Check sheet for the modelled part. Datum: model origin and axes. Units: mm. Face numbers are marked on the shaded views. Round coordinates to 2 decimals unless told otherwise and drop trailing zeros. Write each loop counter-clockwise with the first axis right and the second up, starting at its lowest first coordinate (ties: lowest second). Pieces come first, ordered by that corner, then holes. Notation, with made-up numbers: (62, -27.75) -> (110, -27.75) arc R17 ccw to (110, -2.75) -> close; hole circle Ø10 at (51.25, 13). An arc over 180 degrees is marked (long way). One line per item, written item: value.
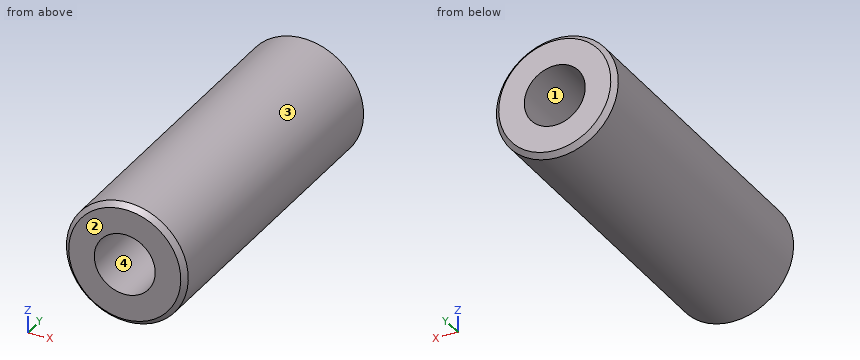
from build123d import *

# Parameters (mm, degrees)
SKETCH_1_R             = 2.5
EXTRUDE_1_DEPTH        = 6.9
HOLE_WIZARD_M3_1_D     = 2.5
HOLE_WIZARD_M3_1_DEPTH = 6.5
HOLE_WIZARD_M3_1_TIP   = 0.751075774
HOLE_WIZARD_M3_2_D     = 2.5
HOLE_WIZARD_M3_2_DEPTH = 6.5
HOLE_WIZARD_M3_2_TIP   = 0.751075774
CHAMFER_1_SIZE         = 0.2


with BuildPart() as part:
    # 草图1 → 凸台-拉伸1 (new, symmetric)
    with BuildSketch(Plane(origin=(0, 0, 0), x_dir=(1, 0, 0), z_dir=(0, 1, 0))):
        with Locations(Location((0, 0, 0), (0, 0, 90))):
            Circle(SKETCH_1_R)
    extrude(amount=EXTRUDE_1_DEPTH, both=True)

    # M3 螺纹孔1
    with Locations(Plane(origin=(0, 6.9, 0), x_dir=(1, 0, 0), z_dir=(0, 1, 0))):
        with Locations((0, 0)):
            Hole(HOLE_WIZARD_M3_1_D / 2, depth=HOLE_WIZARD_M3_1_DEPTH)
            with Locations((0, 0, -(HOLE_WIZARD_M3_1_DEPTH + HOLE_WIZARD_M3_1_TIP / 2))):  # 118° drill point
                Cone(0, HOLE_WIZARD_M3_1_D / 2, HOLE_WIZARD_M3_1_TIP, mode=Mode.SUBTRACT)

    # M3 螺纹孔2
    with Locations(Plane(origin=(0, -6.9, 0), x_dir=(-1, 0, 0), z_dir=(0, -1, 0))):
        with Locations((0, 0)):
            Hole(HOLE_WIZARD_M3_2_D / 2, depth=HOLE_WIZARD_M3_2_DEPTH)
            with Locations((0, 0, -(HOLE_WIZARD_M3_2_DEPTH + HOLE_WIZARD_M3_2_TIP / 2))):  # 118° drill point
                Cone(0, HOLE_WIZARD_M3_2_D / 2, HOLE_WIZARD_M3_2_TIP, mode=Mode.SUBTRACT)

    # 倒角1
    chamfer_1_edges = [part.edges().sort_by_distance(p)[0] for p in [
        (0, -6.9, 2.5),
        (0, 6.9, 2.5),
    ]]
    chamfer(chamfer_1_edges, length=CHAMFER_1_SIZE)


solid = part.part
Item 1: Material ranges on line 1 along Z through (x, y) = (0.1, -4); line 2 along X through (y, z) = (-5, 0.15); line 3 along Z through (x, y) = (-0.75, -2), recorded low to high.
Result set:
line 1: -2.5 to -1.25, 1.25 to 2.5
line 2: -2.5 to -1.24, 1.24 to 2.5
line 3: -2.38 to -1, 1 to 2.38
Item 2: Release check for a two-part mould opening along Z. For the marked faces 1, 2, 3 and 4 record: pulls with the +Z half, pulls with the -Z half, needs draft (parallel to the pull), parting line crosses it, or undercut.
Result set:
face 1: undercut
face 2: needs draft
face 3: parting line crosses it
face 4: undercut
Item 3: Sectioned sample at C-C (y = -5.25). Enter the section's corners in (x, z), then the cut area to 3 significant figures.
Result set:
outline: circle Ø5 at (0, 0); hole circle Ø2.5 at (0, 0)
area: 14.7 mm^2
Item 4: Sectioned sample at A-A (x = 0). Enter the section's corners in (y, z), then the cut area to 3 significant figures.
Result set:
outline: (-6.9, -2.3) -> (-6.7, -2.5) -> (6.7, -2.5) -> (6.9, -2.3) -> (6.9, -1.25) -> (0.4, -1.25) -> (0, -0.58) -> (-0.4, -1.25) -> (-6.9, -1.25) -> close; (-6.9, 1.25) -> (-0.4, 1.25) -> (0, 0.58) -> (0.4, 1.25) -> (6.9, 1.25) -> (6.9, 2.3) -> (6.7, 2.5) -> (-6.7, 2.5) -> (-6.9, 2.3) -> close
area: 35.0 mm^2
Item 5: Depth check by flat-ended pin: pin 1 (1.5 mm diameter, centred on y = 3.5, z = -1.5, fed in from +X); pin 2 (2 mm diameter, centred on x = 0, z = 0, fed in from -Y). Enter the tip coordinate at first touch or a pass-through.
Result set:
pin 1: x = 2.38
pin 2: y = -0.25
Item 6: Sectioned sample at B-B (z = 0). Enter the section's corners in (x, y).
Result set:
outline: (-2.5, -6.7) -> (-2.3, -6.9) -> (-1.25, -6.9) -> (-1.25, -0.4) -> (-0.58, 0) -> (-1.25, 0.4) -> (-1.25, 6.9) -> (-2.3, 6.9) -> (-2.5, 6.7) -> close; (0.58, 0) -> (1.25, -0.4) -> (1.25, -6.9) -> (2.3, -6.9) -> (2.5, -6.7) -> (2.5, 6.7) -> (2.3, 6.9) -> (1.25, 6.9) -> (1.25, 0.4) -> close
